Read the model definition and answer for the solid it produces. Units are mm, in the model's axes. Face numbers are marked on the shaded views. A direction names the side the tool comes from. Coordinates: 2 decimals unless noted, no trailing zeros. Write each loop counter-clockwise with the first axis right and the second up, starting at its lowest first coordinate (ties: lowest second). Pieces come first, ordered by that corner, then holes. Notation, with made-up numbers: M -19.75,-14.75 L 36.25,-14.75 A8 cw 36.25,-1.75 Z; hole C -18.75,28 d7. An arc over 180 degrees is marked long. Write item = value, one per line.
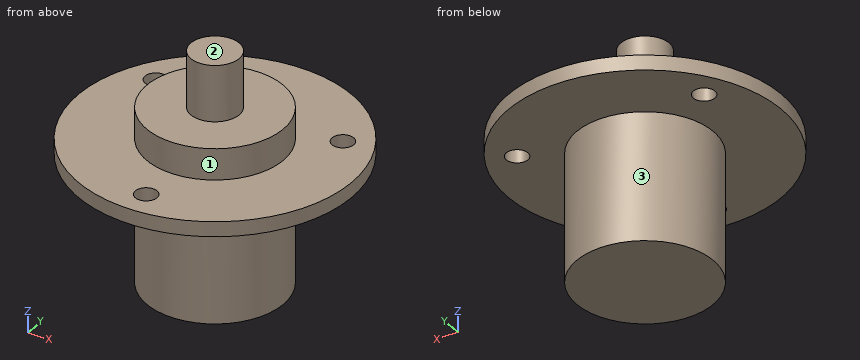
from build123d import *

# Parameters (mm, degrees)
ESQUISSE1_R             = 22
BOSS_EXTRU_1_DEPTH      = 2.4
ESQUISSE1_3_R           = 11
BOSS_EXTRU_2_DEPTH      = 7.4
BOSS_EXTRU_2_DEPTH_BACK = 20.6
ESQUISSE1_4_R           = 3.9
BOSS_EXTRU_3_DEPTH      = 16.4
ESQUISSE1_5_R           = 1.75
ENL_V_MAT_EXTRU_1_DEPTH = 17.4


with BuildPart() as part:
    # Esquisse1 → Boss.-Extru.1 (new body)
    with BuildSketch(Plane.XY):
        Circle(ESQUISSE1_R)
    extrude(amount=BOSS_EXTRU_1_DEPTH)

    # Esquisse1_3 → Boss.-Extru.2 (add, two sides)
    with BuildSketch(Plane.XY) as boss_extru_2_sk:
        Circle(ESQUISSE1_3_R)
    extrude(amount=BOSS_EXTRU_2_DEPTH)
    extrude(boss_extru_2_sk.sketch, amount=-BOSS_EXTRU_2_DEPTH_BACK)

    # Esquisse1_4 → Boss.-Extru.3 (add)
    with BuildSketch(Plane.XY):
        Circle(ESQUISSE1_4_R)
    extrude(amount=BOSS_EXTRU_3_DEPTH)

    # Esquisse1_5 → Enl_v. mat.-Extru.1 (cut, through all)
    with BuildSketch(Plane.XY):
        with Locations((15.155444566, 8.75)):
            Circle(ESQUISSE1_5_R)
        with Locations((-15.155444566, 8.75)):
            Circle(ESQUISSE1_5_R)
        with Locations((0, -17.5)):
            Circle(ESQUISSE1_5_R)
    extrude(amount=ENL_V_MAT_EXTRU_1_DEPTH, mode=Mode.SUBTRACT)


solid = part.part
Item 1: Consider line 1 along Y through (x, z) = (0, 1.7); line 2 along Z through (x, y) = (5.5, -5); line 3 along Z through (x, y) = (7.5, 17). Determine where each line is inside the solid, lowest interval first. Write a range as from..to.
Worked answers:
line_1 = -22..-19.25, -15.75..22
line_2 = -20.6..7.4
line_3 = 0..2.4
Item 2: Flat-ended cylindrical pins translate along their axes: pin 1 (5 mm diameter, centred on y = 16.5, z = 4, fed in from -X); pin 2 (8 mm diameter, centred on x = 17, y = 5.5, fed in from +Z); pin 3 (3 mm diameter, centred on x = 10, z = 5.5, fed in from -Y); pin 4 (17.5 mm diameter, centred on x = 4.5, y = 1.5, fed in from +Z). Find the tip coordinate at first contact, or state that the pin passes through.
Worked answers:
pin_1 = -16.48
pin_2 = 2.4
pin_3 = -6.98
pin_4 = 16.4
Item 3: Find section D-D (y = 8.75). Determine the outline of the cut face in (x, z).
Worked answers:
outline = M -20.19,0 L -16.91,0 L -16.91,2.4 L -20.19,2.4 Z; M -13.41,0 L -6.67,0 L -6.67,-20.6 L 6.67,-20.6 L 6.67,0 L 13.41,0 L 13.41,2.4 L 6.67,2.4 L 6.67,7.4 L -6.67,7.4 L -6.67,2.4 L -13.41,2.4 Z; M 16.91,0 L 20.19,0 L 20.19,2.4 L 16.91,2.4 Z
Item 4: Which of the six approach directions +Z, -Z, +X, -X, +Y, -Y give full straight-line access (tool end or side, diameter ignored) to the marked faces 1, 2 and 3?
Worked answers:
face_1 = +Z
face_2 = +Z, +X, -X, +Y, -Y
face_3 = -Z
Item 5: Find section A-A (x = 0). Determine the outline of the cut face in (y, z).
Worked answers:
outline = M -22,0 L -19.25,0 L -19.25,2.4 L -22,2.4 Z; M -15.75,0 L -11,0 L -11,-20.6 L 11,-20.6 L 11,0 L 22,0 L 22,2.4 L 11,2.4 L 11,7.4 L 3.9,7.4 L 3.9,16.4 L -3.9,16.4 L -3.9,7.4 L -11,7.4 L -11,2.4 L -15.75,2.4 Z
Item 6: Find section C-C (y = 0). Determine the outline of the cut face in (x, z), and give its area (3 significant figures).
Worked answers:
outline = M -22,0 L -11,0 L -11,-20.6 L 11,-20.6 L 11,0 L 22,0 L 22,2.4 L 11,2.4 L 11,7.4 L 3.9,7.4 L 3.9,16.4 L -3.9,16.4 L -3.9,7.4 L -11,7.4 L -11,2.4 L -22,2.4 Z
area = 739 mm²
Item 7: Find section B-B (y = -17.5). Determine the outline of the cut face in (x, z), and give its area (3 significant figures).
Worked answers:
outline = M -13.33,0 L -1.75,0 L -1.75,2.4 L -13.33,2.4 Z; M 1.75,0 L 13.33,0 L 13.33,2.4 L 1.75,2.4 Z
area = 55.6 mm²
